Input: part model. Units: mm. Frame: model coordinates. Give positions to 0.01 mm unless a question says otherwise; leave off trailing zeros. Order: outer loops, then holes, each group sorted by start corner. A loop starts at its lowest first (then second) coordinate and runs counter-clockwise, first axis right, second up. Notation, with made-up numbers: (86.5, 73) -> (103.5, 73) arc R21 ccw to (103.5, 95) -> close; hole circle Ø2 at (89, 76). An arc over 180 degrees is marked (long way). Use a Markdown table: item, result. Add a question column.
from build123d import *

# Parameters (mm, degrees)
SKETCH_1_W                  = 300
SKETCH_1_H                  = 30
EXTRUDE_1_DEPTH             = 5
CHAMFER_1_SIZE              = 1
HOLE_WIZARD_M3_1_D          = 3.2
M3X0_5_1_D                  = 2.5
M4X0_7_1_D                  = 3.3
M4X0_7_2_D                  = 3.3
PATTERN_LINEAR_1_COUNT      = 6
PATTERN_LINEAR_1_PITCH      = 25
PATTERN_LINEAR_1_COL_COUNT  = 7
PATTERN_LINEAR_1_COL_PITCH  = 25
EXTRUDE_3_DEPTH             = 5
SKETCH_13_R                 = 2.6
CUT_EXTRUDE_2_DEPTH         = 161.542829177
HOLE_WIZARD_M2_1_D          = 2.2
M4X0_7_3_D                  = 3.3
HOLE_WIZARD_M4_1_D          = 4.3
M3X0_5_2_D                  = 2.5
CUT_EXTRUDE_3_DEPTH         = 161.542829177
CUT_EXTRUDE_3_DEPTH_BACK    = 161.542829177
SKETCH_25_W                 = 15
SKETCH_25_H                 = 8
FILLET_1_R                  = 1
SKETCH_26_W                 = 30
SKETCH_26_H                 = 5
EXTRUDE_4_DEPTH             = 30
SKETCH_27_R                 = 1.65
CUT_EXTRUDE_4_DEPTH         = 174.476223155
PATTERN_LINEAR_2_COUNT      = 2
PATTERN_LINEAR_2_PITCH      = 20
PATTERN_LINEAR_2_COUNT_DIR2 = 3
PATTERN_LINEAR_2_PITCH_DIR2 = 10
FILLET_2_R                  = 5


with BuildPart() as part:
    # 草圖1 → 填料-伸長1 (new body)
    with BuildSketch(Plane.XY):
        Rectangle(SKETCH_1_W, SKETCH_1_H)
    extrude(amount=EXTRUDE_1_DEPTH)

    # 導角1
    chamfer_1_edges = [part.edges().sort_by_distance(p)[0] for p in [
        (150, -15, 2.5),
        (-150, -15, 2.5),
        (-150, 15, 2.5),
        (150, 15, 2.5),
    ]]
    chamfer(chamfer_1_edges, length=CHAMFER_1_SIZE)

    # M3 餘隙孔1 (through all)
    with Locations(Plane.XY.offset(5)):
        with Locations((20, -10), (20, 10), (0, -10), (0, 10)):
            Hole(HOLE_WIZARD_M3_1_D / 2)

    # M3x0.5 螺紋孔1 (through all)
    with Locations(Plane.XY.offset(5)):
        with Locations((-12.5, 0)):
            m3x0_5_1 = Hole(M3X0_5_1_D / 2)

    # M4x0.7 螺紋孔1 (through all)
    with Locations(Plane.XY.offset(5)):
        with Locations((80, 10), (50, -10), (50, 10), (80, -10), (65, 10), (65, -10)):
            Hole(M4X0_7_1_D / 2)

    # M4x0.7 螺紋孔2 (through all)
    with Locations(Plane.XY.offset(5)):
        with Locations((-126, 10), (-126, -10)):
            m4x0_7_2 = Hole(M4X0_7_2_D / 2)

    # 直線複製排列1: M3x0.5 螺紋孔1 ×6
    with Locations(*[(-i * PATTERN_LINEAR_1_PITCH, 0, 0) for i in range(1, PATTERN_LINEAR_1_COUNT)]):
        add(m3x0_5_1, mode=Mode.SUBTRACT)

    # 直線複製排列1 col: M3x0.5 螺紋孔1 ×7
    with Locations(*[(i * PATTERN_LINEAR_1_COL_PITCH, 0, 0) for i in range(1, PATTERN_LINEAR_1_COL_COUNT)]):
        add(m3x0_5_1, mode=Mode.SUBTRACT)

    # 鏡射1: M4x0.7 螺紋孔2 across plane
    add(m4x0_7_2.mirror(Plane(origin=(0, 0, 0), x_dir=(0, 0, 1), z_dir=(1, 0, 0))), mode=Mode.SUBTRACT)

    # 草圖16 → 填料-伸長3 (add, through all)
    with BuildSketch(Plane.XY):
        with BuildLine():
            Line((-20, 15), (44, 15))
            Line((44, 15), (44, 57))
            Line((44, 57), (0, 57))
            ThreePointArc((0, 57), (-14.142135624, 51.142135624), (-20, 37))
            Line((-20, 37), (-20, 15))
        make_face()
    extrude(amount=EXTRUDE_3_DEPTH)

    # 草圖13 → 除料-伸長2 (cut, through all)
    with BuildSketch(Plane.XY):
        with Locations(Location((34, 24.8, 0), (0, 0, 180))):
            Circle(SKETCH_13_R)
    extrude(amount=CUT_EXTRUDE_2_DEPTH, mode=Mode.SUBTRACT)

    # M2 餘隙孔1 (through all)
    with Locations(Plane.XY.offset(5)):
        with Locations((29, 24.8), (39, 24.8)):
            Hole(HOLE_WIZARD_M2_1_D / 2)

    # M4x0.7 螺紋孔3 (through all)
    with Locations(Plane.XY.offset(5)):
        with Locations((15, 22), (-15, 22)):
            Hole(M4X0_7_3_D / 2)

    # M4 餘隙孔1 (through all)
    with Locations(Plane.XY.offset(5)):
        with Locations((-26, -10), (-26, 10), (-50, -10), (-50, 10)):
            Hole(HOLE_WIZARD_M4_1_D / 2)

    # M3x0.5 螺紋孔2 (through all)
    with Locations(Plane.XY.offset(5)):
        with Locations((33, 53), (33, 45)):
            Hole(M3X0_5_2_D / 2)

    # 草圖25 → 除料-伸長3 (cut, two sides: drawn at the far end of the back side and taken through both)
    with BuildSketch(Plane.XY.offset(5).offset(-CUT_EXTRUDE_3_DEPTH_BACK)):
        with Locations((34, 37)):
            Rectangle(SKETCH_25_W, SKETCH_25_H)
    extrude(amount=CUT_EXTRUDE_3_DEPTH + CUT_EXTRUDE_3_DEPTH_BACK, mode=Mode.SUBTRACT)

    # 圓角1
    fillet_1_edges = [part.edges().sort_by_distance(p)[0] for p in [
        (41.5, 41, 2.5),
        (41.5, 33, 2.5),
        (26.5, 33, 2.5),
        (26.5, 41, 2.5),
    ]]
    fillet(fillet_1_edges, radius=FILLET_1_R)

    # 草圖26 → 填料-伸長4 (add)
    with BuildSketch(Plane(origin=(0, 57, 0), x_dir=(1, 0, 0), z_dir=(0, 1, 0))):
        with Locations((29, -2.5)):
            Rectangle(SKETCH_26_W, SKETCH_26_H)
    extrude(amount=EXTRUDE_4_DEPTH)

    # 草圖27 → 除料-伸長4 (cut, through all)
    with BuildSketch(Plane.XY.offset(5)):
        with Locations((19, 82)):
            Circle(SKETCH_27_R)
    cut_extrude_4 = extrude(amount=-CUT_EXTRUDE_4_DEPTH, mode=Mode.SUBTRACT)

    # 直線複製排列2: Cut-Extrude 4 2 × 3
    with Locations(*[(i * PATTERN_LINEAR_2_PITCH, -j * PATTERN_LINEAR_2_PITCH_DIR2, 0) for i in range(PATTERN_LINEAR_2_COUNT) for j in range(PATTERN_LINEAR_2_COUNT_DIR2) if (i, j) != (0, 0)]):
        add(cut_extrude_4, mode=Mode.SUBTRACT)

    # 圓角2
    fillet_2_edges = [part.edges().sort_by_distance(p)[0] for p in [
        (44, 87, 2.5),
        (14, 87, 2.5),
    ]]
    fillet(fillet_2_edges, radius=FILLET_2_R)


solid = part.part
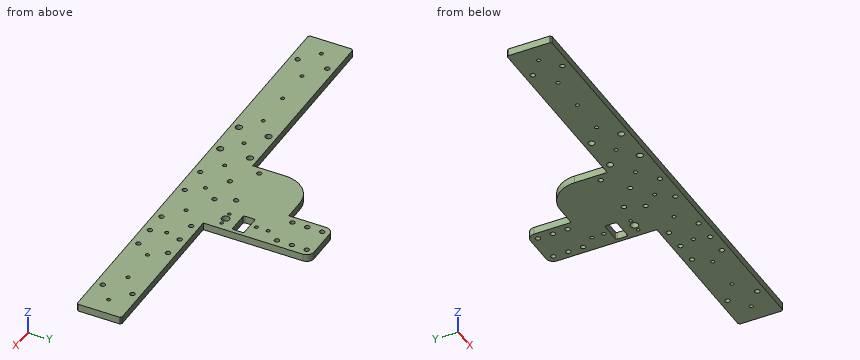
Q1. Section query B-B (z = 4.15). Give the number of separate pieces and of enclosed holes in the cut face, plus the area to 3 significant figures.
Q2. Ray query, line 1 (Y direction, x = 51.5, z = 2); line 2 (X direction, y = 18.5, z = 4.5); line 3 (X direction, y = 37, z = 0.3). Return the intervals inside material, ascending.
Q3. Section query A-A (x = -67.5). Return loops of the section in (y, z).
Q4. First-contact query: pin 1 (1.5 mm diameter, centred on y = 74, z = 2, fed in from -X); pin 2 (2.5 mm diameter, centred on y = 22.5, z = 2, fed in from -X); pin 3 (1.5 mm diameter, centred on y = 37, z = 2.5, fed in from +X). Flat tips, straight axial feed; report the tip coordinate or a pass-through.
Solution:
| question | item | result |
|---|---|---|
| 1 | separate pieces | 1 |
| 1 | enclosed holes | 44 |
| 1 | area | 12,000 mm² |
| 2 | line 1 | y = -15 to -10.69, -9.31 to 9.31, 10.69 to 15 |
| 2 | line 2 | x = -20 to 44 |
| 2 | line 3 | x = -20 to 26.5, 41.5 to 44 |
| 3 | outline | (-15, 0) -> (15, 0) -> (15, 5) -> (-15, 5) -> close |
| 4 | pin 1 | stops at x = 14 |
| 4 | pin 2 | stops at x = -20 |
| 4 | pin 3 | stops at x = 44 |
